Can you work these out from the drawing? Everything is in mm from the part's minimum corner. A direction names the side the tool comes from. Round coordinates to 2 decimals unless told otherwise and drop trailing zeros. Loops run counter-clockwise (first coordinate to the right, second up) from the corner with the lowest first, then second, coordinate; pieces in that order, holes last. Notation, with made-up numbers: M 31.25,-18.5 L 83.25,-18.5 A18 ccw 83.25,-5.5 Z; hole C -28,64.5 d9. An arc over 180 degrees is marked long. Answer in a Markdown table with one row per item.
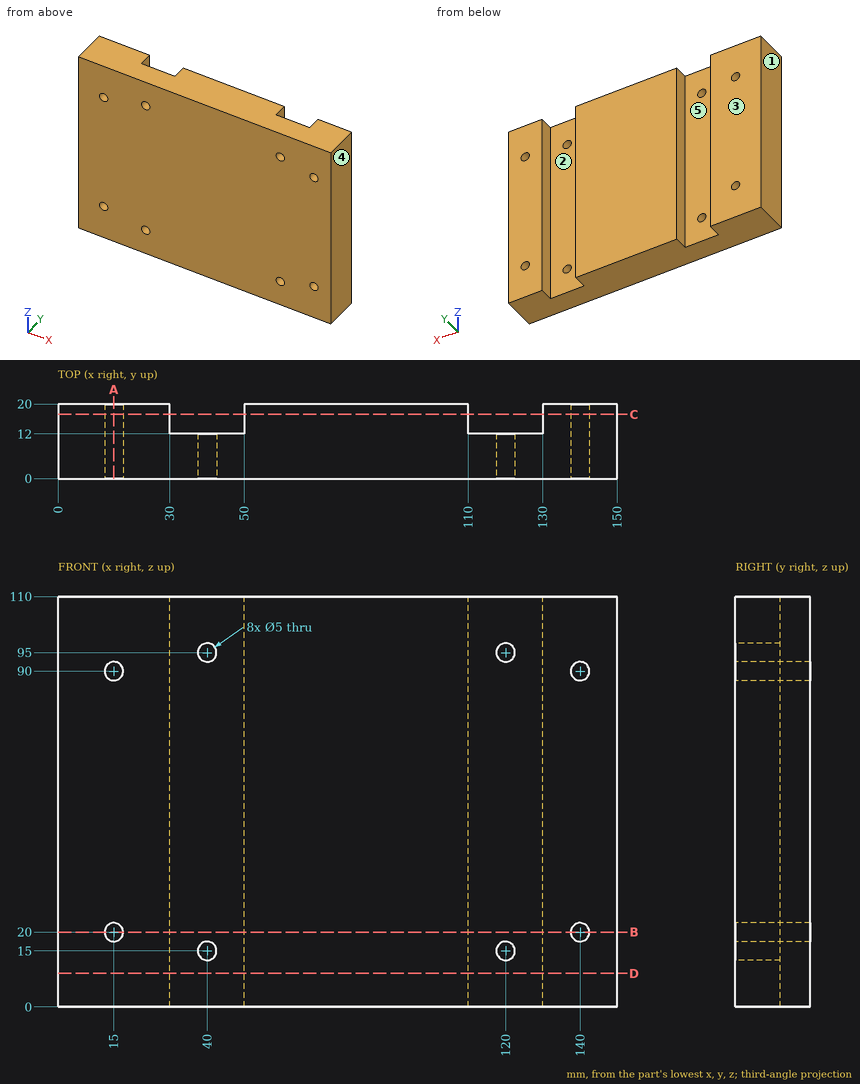
1) I want a section at B-B, the plane z = 20. Please give me the cut outline in (x, y).
Computed:
| item | result |
|---|---|
| outline | M 0,0 L 12.5,0 L 12.5,20 L 0,20 Z; M 17.5,0 L 137.5,0 L 137.5,20 L 130,20 L 130,12 L 110,12 L 110,20 L 50,20 L 50,12 L 30,12 L 30,20 L 17.5,20 Z; M 142.5,0 L 150,0 L 150,20 L 142.5,20 Z |
2) I want a section at C-C, the plane y = 17.25. Please give me the cut outline in (x, z).
Computed:
| item | result |
|---|---|
| outline | M 0,0 L 30,0 L 30,110 L 0,110 Z; M 50,0 L 110,0 L 110,110 L 50,110 Z; M 130,0 L 150,0 L 150,110 L 130,110 Z; hole C 15,20 d5; hole C 15,90 d5; hole C 140,20 d5; hole C 140,90 d5 |
3) Will this pin go through, and if not, where does the flat tip stop? P1, Ø6, axis at x = 43, z = 48, coming from the +Y side.
Computed:
| item | result |
|---|---|
| P1 | stops at y = 12 |
4) I want a section at A-A, the plane x = 15. Please give me the cut outline in (y, z).
Computed:
| item | result |
|---|---|
| outline | M 0,0 L 20,0 L 20,17.5 L 0,17.5 Z; M 0,22.5 L 20,22.5 L 20,87.5 L 0,87.5 Z; M 0,92.5 L 20,92.5 L 20,110 L 0,110 Z |
5) Which directions (+Z, -Z, +X, -X, +Y, -Y) give clear straight access to the entire face, cutting with the end or side of a thin tool? Please do the marked faces 4 and 5.
Computed:
| item | result |
|---|---|
| face 4 | +Z, -Z, +X, +Y, -Y |
| face 5 | +Z, -Z, +Y |
6) I want a section at D-D, the plane z = 9. Please give me the cut outline in (x, y), plus the area to 3 significant figures.
Computed:
| item | result |
|---|---|
| outline | M 0,0 L 150,0 L 150,20 L 130,20 L 130,12 L 110,12 L 110,20 L 50,20 L 50,12 L 30,12 L 30,20 L 0,20 Z |
| area | 2,680 mm² |
7) If we mould it in two halves opening along X, with no side actions, what happens to the marked faces 1, 2 and 3? For each: released by +X, released by -X, zero draft, split by the parting line, or undercut.
Computed:
| item | result |
|---|---|
| face 1 | released by -X |
| face 2 | undercut |
| face 3 | zero draft |
8) I need wall thicknesses on line 1 (X direction, y = 12.25, z = 75); line 2 (Z direction, x = 15, y = 11); line 3 (X direction, y = 9.5, z = 90). Which ranges of each line are inside material? Lowest first, please.
Computed:
| item | result |
|---|---|
| line 1 | x = 0 to 30, 50 to 110, 130 to 150 |
| line 2 | z = 0 to 17.5, 22.5 to 87.5, 92.5 to 110 |
| line 3 | x = 0 to 12.5, 17.5 to 137.5, 142.5 to 150 |
